Read the model definition and answer for the solid it produces. Units are mm, in the model's axes. A direction names the side the tool comes from. Coordinates: 2 decimals unless noted, no trailing zeros. Order: outer loops, then holes, each group sorted by start corner. A loop starts at its lowest first (then second) coordinate and runs counter-clockwise, first axis right, second up.
from build123d import *

# Parameters (mm, degrees)
F1_DEPTH = 31.75
F3_DEPTH = 12.7
F5_DEPTH = 12.7


with BuildPart() as f1:
    # F0 (on Top) → F1 (new body)
    with BuildSketch(Plane.XY):
        Polygon((18.381578, 44.45), (-19.718422, 44.45), (-19.718422, 25.4), (-7.018422, 25.4), (-7.018422, 0), (5.681578, 0), (5.681578, 25.4), (18.381578, 25.4), align=None)
    extrude(amount=F1_DEPTH)

    # F2 (on face) → F3 (join)
    with BuildSketch(Plane.YZ.offset(5.681578)):
        Polygon((12.7, 0), (25.4, 0), (25.4, 31.75), align=None)
    extrude(amount=F3_DEPTH)

    # F4 (on face) → F5 (join)
    with BuildSketch(Plane.YZ.offset(5.681578)):
        Polygon((-12.7, 0), (0, 0), (0, 31.75), align=None)
    extrude(amount=-F5_DEPTH)


solid = f1.part
Q1. Straight lines are drawn through the part: L1, parallel to Y at x = -7.5, z = 23; L2, parallel to X at y = 9, z = 17.5; L3, parallel to X at y = 17.5, z = 8.5. For each, find the intervals that lie inside material, in ascending order.
Q2. Each of these flat-tipped pins is pushed along its axis until it touches: P1, Ø16, axis at y = 1.5, z = 14, coming from the +X side; P2, Ø6.5, axis at x = -11.5, z = 11.5, coming from the -Y side; P3, Ø3, axis at x = 1.5, y = -6.5, coming from the +Z side. Where does it stop, or does it pass through?
Q3. The part is cut by section A-A, the plane z = 4.5. Determine the outline of the cut face in (x, y).
Q4. The part is cut by section C-C, the plane x = 2.5. Determine the outline of the cut face in (y, z).
Q5. The part is cut by section D-D, the plane z = 14.5. Determine the outline of the cut face in (x, y).
Q6. Which of the six approach directions +Z, -Z, +X, -X, +Y, -Y give full straight-line access (tool end or side, diameter ignored) to faces 1 (the flat face through (-13, 25.4, 16)), 2 (the flat face through (5.682, 6, 16)), 3 (the flat face through (0, 44.45, 16))?
Q7. The part is cut by section B-B, the plane y = 20. Determine the outline of the cut face in (x, z), then the cut area to 3 significant figures.
Computed values:
1. L1: y = 25.4 to 44.45
1. L2: x = -7.02 to 5.68
1. L3: x = -7.02 to 18.38
2. P1: stops at x = 5.68
2. P2: stops at y = 25.4
2. P3: stops at z = 19.25
3. outline: (-19.72, 25.4) - (-7.02, 25.4) - (-7.02, -10.9) - (5.68, -10.9) - (5.68, 14.5) - (18.38, 14.5) - (18.38, 44.45) - (-19.72, 44.45) - close
4. outline: (-12.7, 0) - (44.45, 0) - (44.45, 31.75) - (0, 31.75) - close
5. outline: (-19.72, 25.4) - (-7.02, 25.4) - (-7.02, -6.9) - (5.68, -6.9) - (5.68, 18.5) - (18.38, 18.5) - (18.38, 44.45) - (-19.72, 44.45) - close
6. face 1: +Z, -Z, -X, -Y
6. face 2: +Z, +X, -Y
6. face 3: +Z, -Z, +X, -X, +Y
7. outline: (-7.02, 0) - (18.38, 0) - (18.38, 18.25) - (5.68, 18.25) - (5.68, 31.75) - (-7.02, 31.75) - close
7. area: 635 mm2
